Check sheet for the modelled part. Datum: model origin and axes. Units: mm. Round coordinates to 2 decimals unless told otherwise and drop trailing zeros. Write each loop counter-clockwise with the first axis right and the second up, starting at its lowest first coordinate (ties: lowest second). Pieces come first, ordered by that corner, then holes. Notation, with made-up numbers: (67, 33.5) -> (107, 33.5) arc R30 cw to (107, 70.5) -> close; hole circle Ø4 at (84, -20.75). An arc over 180 degrees is marked (long way). Use one line per item in the form item = value. Start each with the question number.
```python
from build123d import *

# Parameters (mm, degrees)
F0_R         = 3.225
F0_R_2       = 1.25
F0_R_3       = 4.95
F1_DEPTH     = 4
F2_T1_DEPTH  = 4
F2_T3_DEPTH  = 4
F2_T5_DEPTH  = 19
F2_T7_DEPTH  = 19
F2_T9_DEPTH  = 19
F2_T11_DEPTH = 19
F3_R         = 5


# Not quite as in the source:
# - a fillet or chamfer that OpenCascade refuses, or shapes differently, is made with other operations: its cross-section is extruded or revolved along the edge and cut away or added


with BuildPart() as f1:
    # F0 (on Top) → F1 (new body)
    with BuildSketch(Plane.XY):
        Polygon((60, 10), (60, 30), (-60, 30), (-60, 10), (-57.5, 10), (-57.5, -30), (57.5, -30), (57.5, 10), align=None)
        with Locations((-37.275, -22.475)):
            Circle(F0_R, mode=Mode.SUBTRACT)
        with Locations((-9.95, -18.35)):
            Circle(F0_R_2, mode=Mode.SUBTRACT)
        with Locations((-52.55, -1.95)):
            Circle(F0_R_2, mode=Mode.SUBTRACT)
        with Locations((0, -22.45)):
            Circle(F0_R_3, mode=Mode.SUBTRACT)
        with Locations((9.95, -18.35)):
            Circle(F0_R_2, mode=Mode.SUBTRACT)
        with Locations((37.275, -22.475)):
            Circle(F0_R, mode=Mode.SUBTRACT)
        with Locations((52.55, -1.95)):
            Circle(F0_R_2, mode=Mode.SUBTRACT)
        with Locations((-24.85, 1.6)):
            Circle(F0_R_2, mode=Mode.SUBTRACT)
        with Locations((-41.9, 20.6)):
            Circle(F0_R_2, mode=Mode.SUBTRACT)
        with Locations((-22.475, 22.475)):
            Circle(F0_R, mode=Mode.SUBTRACT)
        with Locations((24.85, 1.6)):
            Circle(F0_R_2, mode=Mode.SUBTRACT)
        with Locations((22.475, 22.475)):
            Circle(F0_R, mode=Mode.SUBTRACT)
        with Locations((41.9, 20.6)):
            Circle(F0_R_2, mode=Mode.SUBTRACT)
    extrude(amount=F1_DEPTH)

    # F2: fillet of radius 3 on 6 edges, made by hand

    # F2_s2 → F2_t1 (join)
    with BuildSketch(Plane.XY):
        with BuildLine():
            ThreePointArc((-60, 10), (-58.2087121525, 8.9784517816), (-57.5, 7.0419601084))
            Line((-57.5, 7.0419601084), (-57.5, 10))
            Line((-57.5, 10), (-60, 10))
        make_face()
    extrude(amount=F2_T1_DEPTH)

    # F2_s4 → F2_t3 (join)
    with BuildSketch(Plane.XY):
        with BuildLine():
            ThreePointArc((60, 10), (58.2087121525, 8.9784517816), (57.5, 7.0419601084))
            Line((57.5, 7.0419601084), (57.5, 10))
            Line((57.5, 10), (60, 10))
        make_face()
    extrude(amount=F2_T3_DEPTH)

    # F2_s6 → F2_t5 (cut)
    with BuildSketch(Plane.XY.offset(-7.5)):
        with BuildLine():
            ThreePointArc((60, 27), (59.1213203436, 29.1213203436), (57, 30))
            Line((57, 30), (60, 30))
            Line((60, 30), (60, 27))
        make_face()
    extrude(amount=F2_T5_DEPTH, mode=Mode.SUBTRACT)

    # F2_s8 → F2_t7 (cut)
    with BuildSketch(Plane.XY.offset(-7.5)):
        with BuildLine():
            ThreePointArc((-60, 27), (-59.1213203436, 29.1213203436), (-57, 30))
            Line((-57, 30), (-60, 30))
            Line((-60, 30), (-60, 27))
        make_face()
    extrude(amount=F2_T7_DEPTH, mode=Mode.SUBTRACT)

    # F2_s10 → F2_t9 (cut)
    with BuildSketch(Plane.XY.offset(-7.5)):
        with BuildLine():
            ThreePointArc((-54.5, -30), (-56.6213203436, -29.1213203436), (-57.5, -27))
            Line((-57.5, -27), (-57.5, -30))
            Line((-57.5, -30), (-54.5, -30))
        make_face()
    extrude(amount=F2_T9_DEPTH, mode=Mode.SUBTRACT)

    # F2_s12 → F2_t11 (cut)
    with BuildSketch(Plane.XY.offset(-7.5)):
        with BuildLine():
            ThreePointArc((57.5, -27), (56.6213203436, -29.1213203436), (54.5, -30))
            Line((54.5, -30), (57.5, -30))
            Line((57.5, -30), (57.5, -27))
        make_face()
    extrude(amount=F2_T11_DEPTH, mode=Mode.SUBTRACT)

    # F3
    f3_edges = [f1.edges().sort_by_distance(p)[0] for p in [
        (-60, 10, 2),
        (60, 10, 2),
    ]]
    fillet(f3_edges, radius=F3_R)


solid = f1.part
```
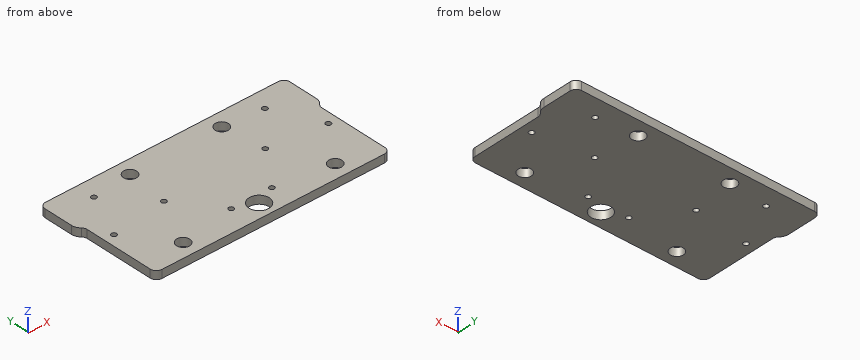
1. Scan lines: probe 1 along Y at (x, z) = (0, 3.25); probe 2 along Y at (x, z) = (-9.95, 1.75); probe 3 along X at (y, z) = (-18.5, 1). Record each from-to range of solid material in increasing order.
2. Sectioned sample at C-C (z = 2.45). Give the number of separate pieces and of enclosed holes in the cut face, and give its area (3 significant figures).
3. Sectioned sample at D-D (y = -7). Enter the section's corners in (x, z).
4. Sectioned sample at B-B (y = 1.6). Enter the section's corners in (x, z).
5. Depth check by flat-ended pin: pin 1 (2 mm diameter, centred on x = -9.95, y = -18.35, fed in from +Z). Enter the tip coordinate at first touch or a pass-through.
6. Sectioned sample at A-A (x = 52.55). Enter the section's corners in (y, z), and give its area (3 significant figures).
Returned:
q1.probe_1 = -30 to -27.4, -17.5 to 30
q1.probe_2 = -30 to -19.6, -17.1 to 30
q1.probe_3 = -57.5 to -11.19, -8.71 to -2.98, 2.98 to 8.71, 11.19 to 57.5
q2.separate_pieces = 1
q2.enclosed_holes = 13
q2.area = 6,750 mm^2
q3.outline = (-57.5, 0) -> (57.5, 0) -> (57.5, 4) -> (-57.5, 4) -> close
q4.outline = (-57.5, 0) -> (-26.1, 0) -> (-26.1, 4) -> (-57.5, 4) -> close; (-23.6, 0) -> (23.6, 0) -> (23.6, 4) -> (-23.6, 4) -> close; (26.1, 0) -> (57.5, 0) -> (57.5, 4) -> (26.1, 4) -> close
q5.pin_1 = through
q6.outline = (-30, 0) -> (-3.2, 0) -> (-3.2, 4) -> (-30, 4) -> close; (-0.7, 0) -> (30, 0) -> (30, 4) -> (-0.7, 4) -> close
q6.area = 230 mm^2
